from build123d import *

# Parameters (mm, degrees)
F0_W     = 76.2
F0_H     = 50.8
F1_DEPTH = 50.8
F3_SIZE  = 25.39999
F4_W     = 6.6249594092
F4_H     = 13.2540166378
F5_DEPTH = 50.801


# Not quite as in the source:
# - a fillet or chamfer is up to 0.001 mm smaller than in the source, because OpenCascade refuses the exact size


with BuildPart() as f1:
    # F0 (on Top) → F1 (new body)
    with BuildSketch(Plane.XY):
        with Locations((38.1, 25.4)):
            Rectangle(F0_W, F0_H)
    extrude(amount=F1_DEPTH)

    # F3 (size 25.4 in the source; OpenCascade refuses exactly that, so slightly less here)
    f3_edges = [f1.edges().sort_by_distance(p)[0] for p in [
        (0, 25.4, 50.8),
        (76.2, 25.4, 50.8),
        (38.1, 0, 50.8),
        (38.1, 50.8, 50.8),
    ]]
    chamfer(f3_edges, length=F3_SIZE)

    # F4 (on face) → F5 (cut, through all)
    with BuildSketch(Plane(origin=(0, 0, 0), x_dir=(1, 0, 0), z_dir=(0, 0, -1))):
        with Locations((42.4170047045, -18.6321474612)):
            Rectangle(F4_W, F4_H)
    extrude(amount=-F5_DEPTH, mode=Mode.SUBTRACT)


solid = f1.part
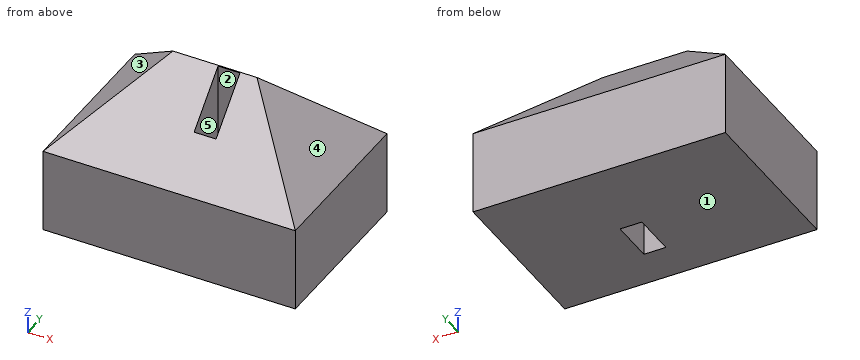
The listing builds one solid part. Answer for the finished solid, in the listing's coordinates (mm). Face numbers are marked on the shaded views. A direction names the side the tool comes from. Give positions to 0.01 mm unless a question says otherwise; leave off trailing zeros. Write each loop counter-clockwise with the first axis right and the second up, starting at its lowest first coordinate (ties: lowest second). Pieces come first, ordered by that corner, then holes.
Item 1: Section B-B, the plane y = 20 is taken. Write down the section's boundary in (x, z), plus the area to 3 significant figures.
Item 2: Find the intervals of material crossed by line 1 along X through (y, z) = (19, 23.5); line 2 along X through (y, z) = (18, 29); line 3 along Y through (x, z) = (41, 32), in increasing order.
Item 3: Section A-A, the plane z = 12 is taken. Write down the section's boundary in (x, y).
Item 4: Section D-D, the plane y = 5.5 is taken. Write down the section's boundary in (x, z).
Item 5: Determine the mould class of the marked faces 3, 4 and 5 for opening direction X: released by +X, released by -X, zero draft, split by the parting line, or undercut.
Item 6: Which of the six approach directions +Z, -Z, +X, -X, +Y, -Y give full straight-line access (tool end or side, diameter ignored) to the marked faces 1 and 2?
Item 7: Flat-ended cylindrical pins translate along their axes: P1, Ø3, axis at x = 14, y = 14.5, coming from the +Z side; P2, Ø12, axis at y = 22, z = 40.5, coming from the +X side; P3, Ø1.5, axis at x = 37, z = 42.5, coming from the -Y side. Find the tip coordinate at first contact, or state that the pin passes through.
Completed:
1. outline: (0, 0) - (39.1, 0) - (39.1, 45.4) - (20, 45.4) - (0, 25.4) - close; (45.73, 0) - (76.2, 0) - (76.2, 25.4) - (56.2, 45.4) - (45.73, 45.4) - close
1. area: 2,760 mm2
2. line 1: x = 0 to 39.1, 45.73 to 76.2
2. line 2: x = 3.6 to 39.1, 45.73 to 72.6
2. line 3: y = 6.6 to 12.01, 25.26 to 44.2
3. outline: (0, 0) - (76.2, 0) - (76.2, 50.8) - (0, 50.8) - close; hole (39.1, 12.01) - (45.73, 12.01) - (45.73, 25.26) - (39.1, 25.26) - close
4. outline: (0, 0) - (76.2, 0) - (76.2, 25.4) - (70.7, 30.9) - (5.5, 30.9) - (0, 25.4) - close
5. face 3: released by -X
5. face 4: released by +X
5. face 5: undercut
6. face 1: -Z, +X, -X, +Y, -Y
6. face 2: +Z, -Z
7. P1: stops at z = 40.68
7. P2: stops at x = 67.1
7. P3: stops at y = 16.35
